Build history of the part. All positions in model axes, mm. A direction names the side the tool comes from. Coordinates: 2 decimals unless noted, no trailing zeros. Order: outer loops, then holes, each group sorted by start corner. A loop starts at its lowest first (then second) coordinate and runs counter-clockwise, first axis right, second up. Notation, with made-up numbers: (60, -20.5) - (71, -20.5) arc R31 cw to (71, 11.5) - close; hole circle Ø6 at (-17.5, 62). An arc over 180 degrees is marked (long way). One line per item, written item: value.
from build123d import *

# Parameters (mm, degrees)
SKETCH1_R           = 10
SKETCH1_R_2         = 0.75
SKETCH1_R_3         = 1.5
BOSS_EXTRUDE1_DEPTH = 2.5
SKETCH5_R           = 4.25
SKETCH5_R_2         = 3
BOSS_EXTRUDE2_DEPTH = 4
SKETCH6_R           = 4.5
CUT_EXTRUDE1_DEPTH  = 0.8
SKETCH7_R           = 3.7
SKETCH7_R_2         = 3.5
BOSS_EXTRUDE3_DEPTH = 0.8
FILLET1_R           = 0.2


with BuildPart() as part:
    # Sketch1 → Boss-Extrude1 (new body)
    with BuildSketch(Plane.XY):
        Circle(SKETCH1_R)
        with Locations((-7, 0)):
            Circle(SKETCH1_R_2, mode=Mode.SUBTRACT)
        with Locations((3.5, 7)):
            Circle(SKETCH1_R_2, mode=Mode.SUBTRACT)
        with Locations((0, 7)):
            Circle(SKETCH1_R_2, mode=Mode.SUBTRACT)
        with Locations((-3.5, 7)):
            Circle(SKETCH1_R_2, mode=Mode.SUBTRACT)
        with Locations((7, -3.5)):
            Circle(SKETCH1_R_2, mode=Mode.SUBTRACT)
        with Locations((7, 0)):
            Circle(SKETCH1_R_2, mode=Mode.SUBTRACT)
        with Locations((7, 3.5)):
            Circle(SKETCH1_R_2, mode=Mode.SUBTRACT)
        with Locations((-3.5, -7)):
            Circle(SKETCH1_R_2, mode=Mode.SUBTRACT)
        with Locations((0, -7)):
            Circle(SKETCH1_R_2, mode=Mode.SUBTRACT)
        with Locations((3.5, -7)):
            Circle(SKETCH1_R_2, mode=Mode.SUBTRACT)
        with Locations((-7, -3.5)):
            Circle(SKETCH1_R_2, mode=Mode.SUBTRACT)
        with Locations((-7, 3.5)):
            Circle(SKETCH1_R_2, mode=Mode.SUBTRACT)
        Circle(SKETCH1_R_3, mode=Mode.SUBTRACT)
    extrude(amount=BOSS_EXTRUDE1_DEPTH)

    # Sketch5 → Boss-Extrude2 (add)
    with BuildSketch(Plane.XY.offset(2.5)):
        Circle(SKETCH5_R)
        Circle(SKETCH5_R_2, mode=Mode.SUBTRACT)
    extrude(amount=BOSS_EXTRUDE2_DEPTH)

    # Sketch6 → Cut-Extrude1 (cut)
    with BuildSketch(Plane(origin=(0, 0, 0), x_dir=(-1, 0, 0), z_dir=(0, 0, -1))):
        Circle(SKETCH6_R)
    extrude(amount=-CUT_EXTRUDE1_DEPTH, mode=Mode.SUBTRACT)

    # Sketch7 → Boss-Extrude3 (add)
    with BuildSketch(Plane(origin=(0, 0, 0.8), x_dir=(-1, 0, 0), z_dir=(0, 0, -1))):
        Circle(SKETCH7_R)
        Circle(SKETCH7_R_2, mode=Mode.SUBTRACT)
    extrude(amount=BOSS_EXTRUDE3_DEPTH)

    # Fillet1
    fillet1_edges = [part.edges().sort_by_distance(p)[0] for p in [
        (-10, 0, 0),
        (-10, 0, 2.5),
        (-4.25, 0, 6.5),
        (4.5, 0, 0),
    ]]
    fillet(fillet1_edges, radius=FILLET1_R)


solid = part.part
1. Band-saw the part on A-A, the plane z = 0.5. Count the separate pieces of the cut face and the enclosed holes in it, and give its area (3 significant figures).
Values found:
separate pieces: 2
enclosed holes: 14
area: 234 mm2
2. Probe line 1 along Y through (x, z) = (0, 0.6); line 2 along Y through (x, z) = (7, 0.65); line 3 along X through (y, z) = (0.5, 2.25). List the from-to ranges inside material, lowest first.
Values found:
line 1: y = -10 to -7.75, -6.25 to -4.5, -3.7 to -3.5, 3.5 to 3.7, 4.5 to 6.25, 7.75 to 10
line 2: y = -7.14 to -4.25, -2.75 to -0.75, 0.75 to 2.75, 4.25 to 7.14
line 3: x = -9.99 to -7.56, -6.44 to -1.41, 1.41 to 6.44, 7.56 to 9.99
3. Two-plate mould, pull along Y, no slides. Class faces 1 (the face through (-7.75, 0.03, 1.23)), 2 (the face through (-4.25, -6.97, 1.23)), 3 (the face through (2.285, 3.584, 4.373)), 4 (the face through (4, -2, 2.5)): pulls with the +Y half, pulls with the -Y half, needs draft (parallel to the pull), parting line crosses it, or undercut.
Values found:
face 1: undercut
face 2: undercut
face 3: parting line crosses it
face 4: needs draft
4. Flat gauge pins, fed straight in: P1, Ø3, axis at x = -1, y = 7.5, coming from the +Z side; P2, Ø2.5, axis at x = 1.5, y = -0.5, coming from the -Z side; P3, Ø2.5, axis at x = 0, y = 0, coming from the +Z side; P4, Ø1.5, axis at x = -0.5, z = 4.5, coming from the +Y side. Where does each tip first touch, or does it go through?
Values found:
P1: stops at z = 2.5
P2: stops at z = 0.8
P3: passes through
P4: stops at y = 4.25
5. Band-saw the part on C-C, the plane z = 5. Give the cut face in (x, y).
Values found:
outline: circle Ø8.5 at (0, 0); hole circle Ø6 at (0, 0)
6. 3-axis set-ups, long thin cutter, end or side, ignore diameter. For faces 5 (the face through (1.3, -1.3, 2.5)), 6 (the face through (2.75, -6.97, 1.23)), 7 (the face through (0.802, -3.612, 0.406)): which of +Z, -Z, +X, -X, +Y, -Y reach the whole face in a straight line?
Values found:
face 5: +Z
face 6: +Z, -Z
face 7: -Z
